Study the drawing (mm; zero at the part's minimum x, y, z) and answer. Coordinates: 2 decimals unless noted, no trailing zeros. Write each loop counter-clockwise with the first axis right and the second up, starting at its lowest first coordinate (ties: lowest second). Pieces come first, ordered by that corner, then holes. Notation, with made-up numbers: M 68,-40 L 114,-40 A31 ccw 114,-13 Z; hole C -11.75,60.5 d10. An arc over 180 degrees is marked long. Answer as CSV lines item,"result". Start each with the question number.
(1) A cutting plane is placed at A-A on z = 94. Give the vertices of the cut face in (x, y), then the cut area to 3 significant figures.
(2) A cutting plane is placed at C-C on x = 30. Give the vertices of the cut face in (y, z) (1 decimal), then the cut area to 3 significant figures.
(3) Find the intervals of material crossed by L1, parallel to X at y = 2.2, z = 94; L2, parallel to Z at x = 19.5, y = 1.6 (1 decimal); L3, parallel to Z at x = 36.5, y = 1.6 (1 decimal), in increasing order. Write a range as [from, to].
(4) A cutting plane is placed at B-B on y = 0.75. Give the vertices of the cut face in (x, z) (1 decimal).
(5) A flat-ended cylindrical pin translates along its axis: P1, Ø4, axis at x = 78.33, z = 6, coming from the +Y side. Find the tip coordinate at first contact, or state that the pin passes through.
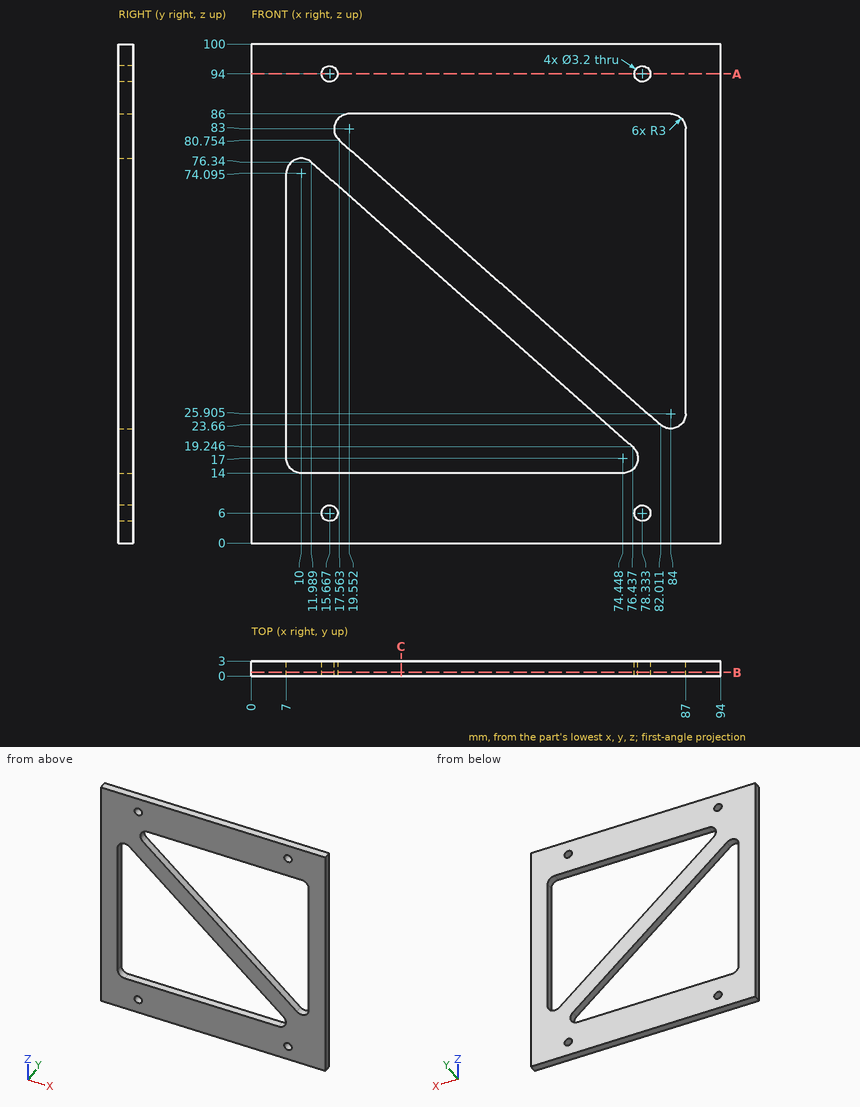
Here are the results:
1,outline,"M 0,0 L 14.07,0 L 14.07,3 L 0,3 Z; M 17.27,0 L 76.73,0 L 76.73,3 L 17.27,3 Z; M 79.93,0 L 94,0 L 94,3 L 79.93,3 Z"
1,area,"263 mm^2"
2,outline,"M 0,0 L 3,0 L 3,14 L 0,14 Z; M 0,60.4 L 3,60.4 L 3,69.7 L 0,69.7 Z; M 0,86 L 3,86 L 3,100 L 0,100 Z"
2,area,"112 mm^2"
3,L1,"x = [0, 14.07], [17.27, 76.73], [79.93, 94]"
3,L2,"z = [0, 14], [69.7, 79], [86, 100]"
3,L3,"z = [0, 14], [54.6, 64], [86, 100]"
4,outline,"M 0,0 L 94,0 L 94,100 L 0,100 Z; hole M 7,17 A3 ccw 10,14 L 74.4,14 A3 ccw 76.4,19.2 L 12,76.3 A3 ccw 7,74.1 Z; hole C 15.7,6 d3.2; hole C 15.7,94 d3.2; hole M 17.6,80.8 L 82,23.7 A3 ccw 87,25.9 L 87,83 A3 ccw 84,86 L 19.6,86 A3 ccw Z; hole C 78.3,6 d3.2; hole C 78.3,94 d3.2"
5,P1,"stops at y = 3"
